Source: CAD feature listing. Evaluate the final solid. Frame: model axes, mm. Round coordinates to 2 decimals unless told otherwise and drop trailing zeros. Loops run counter-clockwise (first coordinate to the right, second up) from the corner with the lowest first, then second, coordinate; pieces in that order, holes last. Notation, with made-up numbers: M 28,-13 L 69,-13 A6 ccw 69,-7 Z; hole C 55,46.5 d8. An arc over 180 degrees is marked long. Answer as a JSON object with one key per item and string values.
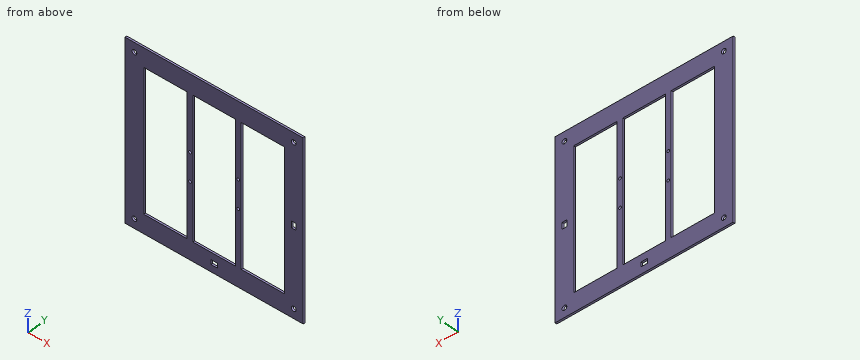
from build123d import *

# Parameters (mm, degrees)
CROQUIS1_W              = 190
CROQUIS1_H              = 190
CROQUIS1_R              = 1.5
CROQUIS1_R_2            = 2.5
CROQUIS1_W_2            = 46.25
CROQUIS1_H_2            = 150
CROQUIS1_W_3            = 45.5
CROQUIS1_W_4            = 5
CROQUIS1_H_3            = 7
CROQUIS1_W_5            = 7
CROQUIS1_H_4            = 5
SALIENTE_EXTRUIR1_DEPTH = 2


with BuildPart() as part:
    # Croquis1 → Saliente-Extruir1 (new body)
    with BuildSketch(Plane(origin=(0, 0, 0), x_dir=(1, 0, 0), z_dir=(0, 1, 0))):
        with Locations((85, 85)):
            Rectangle(CROQUIS1_W, CROQUIS1_H)
        with Locations(Location((59.25, 100, 0), (0, 0, 270))):
            Circle(CROQUIS1_R, mode=Mode.SUBTRACT)
        with Locations(Location((59.25, 70, 0), (0, 0, 270))):
            Circle(CROQUIS1_R, mode=Mode.SUBTRACT)
        with Locations(Location((0, 170, 0), (0, 0, 270))):
            Circle(CROQUIS1_R_2, mode=Mode.SUBTRACT)
        with Locations(Location((0, 0, 0), (0, 0, 270))):
            Circle(CROQUIS1_R_2, mode=Mode.SUBTRACT)
        with Locations(Location((110.75, 100, 0), (0, 0, 90))):
            Circle(CROQUIS1_R, mode=Mode.SUBTRACT)
        with Locations(Location((110.75, 70, 0), (0, 0, 90))):
            Circle(CROQUIS1_R, mode=Mode.SUBTRACT)
        with Locations(Location((170, 0, 0), (0, 0, 90))):
            Circle(CROQUIS1_R_2, mode=Mode.SUBTRACT)
        with Locations(Location((170, 170, 0), (0, 0, 90))):
            Circle(CROQUIS1_R_2, mode=Mode.SUBTRACT)
        with Locations((33.125, 85)):
            Rectangle(CROQUIS1_W_2, CROQUIS1_H_2, mode=Mode.SUBTRACT)
        with Locations((136.875, 85)):
            Rectangle(CROQUIS1_W_2, CROQUIS1_H_2, mode=Mode.SUBTRACT)
        with Locations((85, 85)):
            Rectangle(CROQUIS1_W_3, CROQUIS1_H_2, mode=Mode.SUBTRACT)
        with Locations((170, 85)):
            Rectangle(CROQUIS1_W_4, CROQUIS1_H_3, mode=Mode.SUBTRACT)
        with Locations((85, 170)):
            Rectangle(CROQUIS1_W_5, CROQUIS1_H_4, mode=Mode.SUBTRACT)
    extrude(amount=SALIENTE_EXTRUIR1_DEPTH)


solid = part.part
Item 1: Section B-B on x = 0. Return the cut outline in (y, z).
Answer sheet:
{"outline": "M 0,-180 L 2,-180 L 2,-172.5 L 0,-172.5 Z; M 0,-167.5 L 2,-167.5 L 2,-2.5 L 0,-2.5 Z; M 0,2.5 L 2,2.5 L 2,10 L 0,10 Z"}
Item 2: Section D-D on y = 0.95. Give the number of separate pieces and of enclosed holes in the cut face, then the cut area to 3 significant figures.
Answer sheet:
{"separate pieces": "1", "enclosed holes": "13", "area": "15,200 mm²"}
Item 3: Contact query for a flat-ended pin moving along its axis: pin 1 Ø2.5 at (x, z) = (110.75, -70) entering from +Y. Output: stop coordinate, or through.
Answer sheet:
{"pin 1": "passes through"}
Item 4: Section A-A on z = -170. Return the cut outline in (x, y), then the cut area to 3 significant figures.
Answer sheet:
{"outline": "M -10,0 L -2.5,0 L -2.5,2 L -10,2 Z; M 2.5,0 L 81.5,0 L 81.5,2 L 2.5,2 Z; M 88.5,0 L 167.5,0 L 167.5,2 L 88.5,2 Z; M 172.5,0 L 180,0 L 180,2 L 172.5,2 Z", "area": "346 mm²"}
Item 5: Line query: probe 1 along X at (y, z) = (0.55, -170); probe 2 along X at (y, z) = (0.55, -100); probe 3 along Z at (x, y) = (110.75, 0.85). Output: solid intervals per line, ascending. Write a range as from..to.
Answer sheet:
{"probe 1": "x = -10..-2.5, 2.5..81.5, 88.5..167.5, 172.5..180", "probe 2": "x = -10..10, 56.25..57.75, 60.75..62.25, 107.75..109.25, 112.25..113.75, 160..180", "probe 3": "z = -180..-101.5, -98.5..-71.5, -68.5..10"}
Item 6: Section C-C on x = 38. Return the cut outline in (y, z).
Answer sheet:
{"outline": "M 0,-180 L 2,-180 L 2,-160 L 0,-160 Z; M 0,-10 L 2,-10 L 2,10 L 0,10 Z"}
